Could you check a few things on this model? Use its own coordinates, in mm. A direction names the side the tool comes from. Coordinates: 2 decimals unless noted, no trailing zeros. Loops run counter-clockwise (first coordinate to the right, second up) from the corner with the lowest first, then second, coordinate; pieces in that order, holes last.
from build123d import *

# Parameters (mm, degrees)
F1_DEPTH = 22.225
F2_R     = 5.08
F3_R     = 9.525
F4_R     = 7.14375
F5_DEPTH = 25.4
F6_R     = 7.14375
F7_DEPTH = 25.4
F8_R     = 5.08


with BuildPart() as f1:
    # F0 (on Front) → F1 (new body, symmetric)
    with BuildSketch(Plane.XZ):
        Polygon((-78.60008, 0), (-76.23788, 0), (-37.32508, 0), (108.721218, 146.046298), (108.721218, 184.959098), (108.721218, 187.321298), (102.371218, 187.321298), (102.371218, 184.959098), (102.371218, 148.676554), (-39.955336, 6.35), (-76.23788, 6.35), (-78.60008, 6.35), align=None)
    extrude(amount=F1_DEPTH, both=True)

    # F2
    f2_edges = [f1.edges().sort_by_distance(p)[0] for p in [
        (-39.955336, 0, 6.35),
        (102.371218, 0, 148.676554),
    ]]
    fillet(f2_edges, radius=F2_R)

    # F3
    f3_edges = [f1.edges().sort_by_distance(p)[0] for p in [
        (108.721218, 0, 146.046298),
        (-37.32508, 0, 0),
    ]]
    fillet(f3_edges, radius=F3_R)

    # F4 (on face) → F5 (cut)
    with BuildSketch(Plane.XY.offset(6.35)):
        with Locations((-57.96258, 0)):
            Circle(F4_R)
    extrude(amount=-F5_DEPTH, mode=Mode.SUBTRACT)

    # F6 (on face) → F7 (cut)
    with BuildSketch(Plane(origin=(102.371218, 0, 0), x_dir=(0, -1, 0), z_dir=(-1, 0, 0))):
        with Locations((0, 166.671098)):
            Circle(F6_R)
    extrude(amount=-F7_DEPTH, mode=Mode.SUBTRACT)

    # F8
    f8_edges = [f1.edges().sort_by_distance(p)[0] for p in [
        (108.721218, 0, 187.321298),
        (-78.60008, 0, 0),
    ]]
    fillet(f8_edges, radius=F8_R)


solid = f1.part
1) Imagine slicing it at A-A on y = 0. State how many separate pieces and enclosed holes the cut face has, plus the area to 3 significant figures.
2) For faces 5 (the flat face through (-64, -5, 6.35)), 6 (the flat face through (-50, 0, 0)), which set-ups out of +Z, -Z, +X, -X, +Y, -Y let a thin tool reach every point of the face, with its end or its side?
3) We'd pull the mould along Z, two halves only. Please class faces 1 (the cylindrical face through (105.502, 0.93, 173.754)), 2 (the flat face through (32.183, -0.311, 78.489)), 3 (the cylindrical face through (-65.1, 0.3, 3.2)), 4 (the cylindrical face through (-37.577, -0.311, 0.745)): released by +Z, released by -Z, zero draft, split by the parting line, or undercut.
4) Imagine slicing it at D-D on z = 134.5. List the corners of the cut face in (x, y) for me (3 decimals), plus the area to 3 significant figures.
5) Will these pins go through, and if not, where does the flat tip stop? pin 1 (6 mm diameter, centred on y = -12, z = 57, fed in from +X); pin 2 (2 mm diameter, centred on x = -33, y = -17, fed in from -Z); pin 3 (1 mm diameter, centred on x = -13, y = 0.5, fed in from +Z).
6) Imagine slicing it at C-C on x = -46. List the corners of the cut face in (y, z) for me (3 decimals).
7) If I drill on L1, parallel to Z at x = -42, y = -19.5; L2, parallel to X at y = 8, z = 174; L3, parallel to Z at x = 106, y = 0, over which ranges is the centre line in solid material (lowest first)?
Solved:
1. separate pieces: 3
1. enclosed holes: 0
1. area: 1,610 mm2
2. face 5: +Z, -X, +Y, -Y
2. face 6: -Z, +X, -X, +Y, -Y
3. face 1: undercut
3. face 2: released by +Z
3. face 3: zero draft
3. face 4: released by -Z
4. outline: (88.195, -22.225) - (97.175, -22.225) - (97.175, 22.225) - (88.195, 22.225) - close
4. area: 399 mm2
5. pin 1: stops at x = 22.67
5. pin 2: stops at z = 3.33
5. pin 3: stops at z = 33.81
6. outline: (-22.225, 0) - (22.225, 0) - (22.225, 6.35) - (-22.225, 6.35) - close
7. L1: z = 0 to 6.35
7. L2: x = 102.37 to 108.72
7. L3: z = 143.33 to 159.53, 173.81 to 186.74
